```python
from build123d import *

# Parameters (mm, degrees)
SKETCH1_R           = 59
BOSS_EXTRUDE1_DEPTH = 6
CUT_EXTRUDE4_DEPTH  = 7
CIRPATTERN2_COUNT   = 4
SKETCH4_R           = 10
CUT_EXTRUDE6_DEPTH  = 10
SKETCH5_R           = 14.75
SKETCH5_R_2         = 10
BOSS_EXTRUDE2_DEPTH = 4
CUT_EXTRUDE8_DEPTH  = 6
CUT_EXTRUDE9_START  = -4
CUT_EXTRUDE9_DEPTH  = 2
CIRPATTERN3_COUNT   = 2


with BuildPart() as part:
    # Sketch1 → Boss-Extrude1 (new body)
    with BuildSketch(Plane(origin=(0, 0, 0), x_dir=(1, 0, 0), z_dir=(0, 1, 0))):
        Circle(SKETCH1_R)
    extrude(amount=BOSS_EXTRUDE1_DEPTH)

    # Sketch2_3 → Cut-Extrude4 (cut, through all)
    with BuildSketch(Plane(origin=(0, 6, 0), x_dir=(1, 0, 0), z_dir=(0, 1, 0))):
        with BuildLine():
            Line((-8.984902794, 28.496471002), (-15.610657267, 49.510679451))
            ThreePointArc((-15.610657267, 49.510679451), (-15.369454974, 51.874258292), (-13.485054862, 53.321227437))
            ThreePointArc((-13.485054862, 53.321227437), (0, 55), (13.485054862, 53.321227437))
            ThreePointArc((13.485054862, 53.321227437), (15.369454974, 51.874258292), (15.610657267, 49.510679451))
            Line((15.610657267, 49.510679451), (8.984902794, 28.496471002))
            ThreePointArc((8.984902794, 28.496471002), (7.172866282, 25.967776979), (4.216318041, 25))
            Line((4.216318041, 25), (-4.216318041, 25))
            ThreePointArc((-4.216318041, 25), (-7.172866282, 25.967776979), (-8.984902794, 28.496471002))
        make_face()
    cut_extrude4 = extrude(amount=-CUT_EXTRUDE4_DEPTH, mode=Mode.SUBTRACT)

    # CirPattern2: Cut-Extrude4 ×4 about axis
    cirpattern2_axis = Axis((0, 0, 0), (0, 1, 0))
    for i in range(1, CIRPATTERN2_COUNT):
        add(cut_extrude4.rotate(cirpattern2_axis, i * 360 / CIRPATTERN2_COUNT), mode=Mode.SUBTRACT)

    # Sketch4 → Cut-Extrude6 (cut)
    with BuildSketch(Plane(origin=(0, 6, 0), x_dir=(1, 0, 0), z_dir=(0, 1, 0))):
        Circle(SKETCH4_R)
    extrude(amount=-CUT_EXTRUDE6_DEPTH, mode=Mode.SUBTRACT)

    # Sketch5 → Boss-Extrude2 (add)
    with BuildSketch(Plane(origin=(0, 6, 0), x_dir=(1, 0, 0), z_dir=(0, 1, 0))):
        Circle(SKETCH5_R)
        Circle(SKETCH5_R_2, mode=Mode.SUBTRACT)
    extrude(amount=BOSS_EXTRUDE2_DEPTH)

    # Sketch6 → Cut-Extrude8 (cut)
    with BuildSketch(Plane(origin=(0, 10, 0), x_dir=(1, 0, 0), z_dir=(0, 1, 0))):
        with BuildLine():
            Line((0, 12.5), (0, 10))
            ThreePointArc((0, 10), (3.826834324, 9.238795325), (7.071067812, 7.071067812))
            Line((7.071067812, 7.071067812), (8.838834765, 8.838834765))
            ThreePointArc((8.838834765, 8.838834765), (4.783542905, 11.548494156), (0, 12.5))
        make_face()
    cut_extrude8 = extrude(amount=-CUT_EXTRUDE8_DEPTH, mode=Mode.SUBTRACT)

    # Sketch6_4 → Cut-Extrude9 (cut)
    with BuildSketch(Plane(origin=(0, 10, 0), x_dir=(1, 0, 0), z_dir=(0, 1, 0)).offset(CUT_EXTRUDE9_START)):
        with BuildLine():
            Line((8.838834765, 8.838834765), (7.071067812, 7.071067812))
            ThreePointArc((7.071067812, 7.071067812), (9.238795325, 3.826834324), (10, 0))
            Line((10, 0), (12.5, 0))
            ThreePointArc((12.5, 0), (11.548494156, 4.783542905), (8.838834765, 8.838834765))
        make_face()
    cut_extrude9 = extrude(amount=-CUT_EXTRUDE9_DEPTH, mode=Mode.SUBTRACT)

    # CirPattern3: Cut-Extrude8, Cut-Extrude9 ×2 about axis
    cirpattern3_axis = Axis((0, 0, 0), (0, 1, 0))
    for i in range(1, CIRPATTERN3_COUNT):
        add(cut_extrude8.rotate(cirpattern3_axis, i * 360 / CIRPATTERN3_COUNT), mode=Mode.SUBTRACT)
        add(cut_extrude9.rotate(cirpattern3_axis, i * 360 / CIRPATTERN3_COUNT), mode=Mode.SUBTRACT)


solid = part.part
```
Can you work these out from the model? Positions are in its coordinate system, mm. A direction names the side the tool comes from. Round coordinates to 2 decimals unless told otherwise and drop trailing zeros. Loops run counter-clockwise (first coordinate to the right, second up) from the corner with the lowest first, then second, coordinate; pieces in that order, holes last. Notation, with made-up numbers: (-26, -34.75) -> (29, -34.75) arc R18 ccw to (29, -17.75) -> close; hole circle Ø1 at (56.25, -11). An arc over 180 degrees is marked (long way). One line per item, written item: value. Start each with the question number.
1. If we section it at B-B, the plane x = 36: Write out the boundary of the cut face in (y, z).
2. If we mould it in two halves opening along Z, with no side actions, what happens to faces 3 (the flat face through (-1, 0, 12)), 4 (the cylindrical face through (56.275, 2.958, -17.722)), 5 (the flat face through (-39.151, 3.042, -12.344))? For each: pulls with the +Z half, pulls with the -Z half, needs draft (parallel to the pull), parting line crosses it, or undercut.
3. If we section it at C-C, the plane x = -20: Write out the boundary of the cut face in (y, z), then the cut area to 3 significant figures.
4. For faces 1 (the cylindrical face through (-15.353, 3.042, 51.904)), 2 (the flat face through (3, 10, 10)), which set-ups out of +Z, -Z, +X, -X, +Y, -Y let a thin tool reach every point of the face, with its end or its side?
5. For pin 1 (4 mm diameter, centred on x = -41, y = 5.5, fed in from -Z); pin 2 (5 mm diameter, centred on x = 0.5, y = 3, fed in from -Z); pin 3 (1.5 mm diameter, centred on x = -26.5, z = 20.5, fed in from +Y); pin 4 (10 mm diameter, centred on x = -20.5, z = -19, fed in from -Y), each with a flat end and sliding along its axis, tell me the tip position at first contact or that it passes through.
6. If we section it at D-D, the plane z = 17.5: Write out the boundary of the cut face in (x, y), then the cut area to 3 significant figures.
7. If we section it at A-A, the plane z = -39: Write out the boundary of the cut face in (x, y), then the cut area to 3 significant figures.
8. If I drill on probe 1 along X at (y, z) = (2.65, 0); probe 2 along Y at (x, z) = (16.5, 37.5), over which ranges is the centre line in solid material (lowest first)?
Calculated:
1. outline: (0, -46.74) -> (6, -46.74) -> (6, -11.35) -> (0, -11.35) -> close; (0, 11.35) -> (6, 11.35) -> (6, 46.74) -> (0, 46.74) -> close
2. face 3: needs draft
2. face 4: parting line crosses it
2. face 5: undercut
3. outline: (0, -55.51) -> (6, -55.51) -> (6, 55.51) -> (0, 55.51) -> close
3. area: 666 mm²
4. face 1: +Y, -Y
4. face 2: +Z, -Z, +X, -X, +Y
5. pin 1: stops at z = -44.27
5. pin 2: stops at z = -59
5. pin 3: stops at y = 6
5. pin 4: stops at y = 0
6. outline: (-56.34, 0) -> (56.34, 0) -> (56.34, 6) -> (-56.34, 6) -> close
6. area: 676 mm²
7. outline: (-44.27, 0) -> (-12.3, 0) -> (-12.3, 6) -> (-44.27, 6) -> close; (12.3, 0) -> (44.27, 0) -> (44.27, 6) -> (12.3, 6) -> close
7. area: 384 mm²
8. probe 1: x = -59 to -55, -25 to -10, 10 to 25, 55 to 59
8. probe 2: y = 0 to 6
